For this review, take the finished solid that the model builds, in its own axes (mm). Face numbers are marked on the shaded views. A direction names the side the tool comes from. Give positions to 0.01 mm unless a question says otherwise; leave off trailing zeros. Order: outer loops, then holes, each group sorted by start corner. A loop starts at its lowest first (then second) coordinate and runs counter-clockwise, first axis right, second up.
Item 1: Consider section B-B (x = 0). Give the boundary of the cut face in (y, z), plus the area to 3 significant figures.
Item 2: For P1, Ø4, axis at x = -18.5, z = 0, coming from the -Y side; P2, Ø8, axis at x = 18.5, z = 0, coming from the +Y side; P3, Ø5, axis at x = -12, y = 4.5, coming from the -Z side; P4, Ø1, axis at y = 4, z = -4, coming from the +X side, all flat-tipped, find the tip position at first contact; note any pin that passes through.
Item 3: Consider section C-C (y = 0.5). Give the boundary of the cut face in (x, z).
Item 4: For probe 1 along Z at (x, y) = (0, 4.5); probe 2 along X at (y, z) = (1.25, 0.25); probe 3 along X at (y, z) = (7.5, -5.75), list the stretches that pass through material, from the lowest coordinate up.
Item 5: Consider section D-D (y = 6.25). Give the boundary of the cut face in (x, z), plus the area to 3 significant figures.
Item 6: Consider section A-A (z = 0). Give the boundary of the cut face in (x, y), plus the area to 3 significant figures.
Item 7: Machinability: for the marked faces 1 and 2, which of the approach directions +Z, -Z, +X, -X, +Y, -Y give a long, thin tool a straight path to every point of the face, cutting with its end or side? Answer none if there is none.
Autodesk Inventor part; units mm, degrees
ref_plane "YZ Plane" through (0, 0, 0) normal (1, 0, 0) x (0, 1, 0)
ref_plane "XZ Plane" through (0, 0, 0) normal (0, 1, 0) x (-1, 0, 0)
ref_plane "XY Plane" through (0, 0, 0) normal (0, 0, 1) x (1, 0, 0)
sketch "Sketch1" plane through (0, 0, 0) normal (0, 1, 0) x (-1, 0, 0)
  circle A0 centre (0, 0) radius 13.25
  circle A1 centre (0, 0) radius 4
  dimension "d0" = 26.5
  dimension "d1" = 8
extrude "Extrusion1" add sketch "Sketch1" along normal blind 8.5
sketch "Sketch2" plane through (0, 0, 0) normal (0, -1, 0) x (1, 0, 0)
  circle A0 centre (18.5, 0) radius 2.5
  circle A1 centre (-18.5, 0) radius 2.5
  circle A2 centre (18.5, 0) radius 5.25
  circle A3 centre (-18.5, 0) radius 5.25
  line L0 (20.7703, -4.7337) -> (5.7297, -11.9471)
  circle A4 centre (0, 0) radius 13.25
  line L1 (20.7703, 4.7337) -> (5.7297, 11.9471)
  line L2 (-5.7297, -11.9471) -> (-20.7703, -4.7337)
  line L3 (-5.7297, 11.9471) -> (-20.7703, 4.7337)
  point P0 (0, 18.5)
  point P1 (0, -18.5)
  dimension "d6" = 5
  dimension "d7" = 5
  dimension "d8" = 37
  dimension "d9" = 18.5
  dimension "d10" = 10.5
  dimension "d11" = 10.5
  dimension "d14" = 47.5
extrude "Extrusion2" add sketch "Sketch2" against normal blind 4.5 contours A2 | A2 A4 L1 | L0 A4 A2 | A4 A3 L3 | L2 A3 A4 | A3
properties part number "O_Do_Lan" material "Aluminum 6061-AHC"
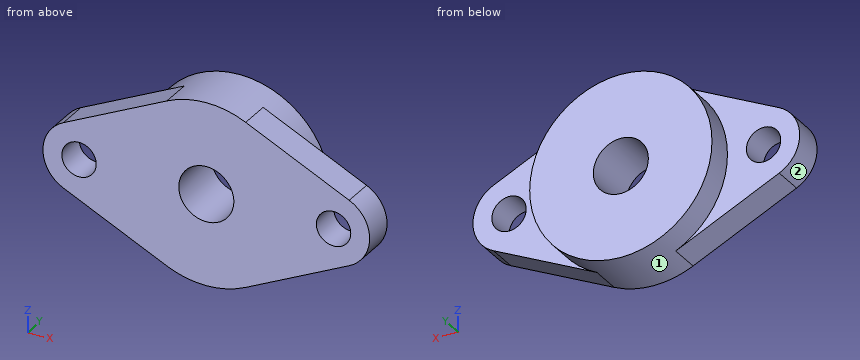
Resolved:
1. outline: (0, -13.25) - (8.5, -13.25) - (8.5, -4) - (0, -4) - close; (0, 4) - (8.5, 4) - (8.5, 13.25) - (0, 13.25) - close
1. area: 157 mm2
2. P1: passes through
2. P2: stops at y = 4.5
2. P3: stops at z = -10.14
2. P4: stops at x = 22.41
3. outline: (-20.77, -4.73) - (-5.73, -11.95) arc R13.25 ccw to (5.73, -11.95) - (20.77, -4.73) arc R5.25 ccw to (20.77, 4.73) - (5.73, 11.95) arc R13.25 ccw to (-5.73, 11.95) - (-20.77, 4.73) arc R5.25 ccw to start; hole circle Ø5 at (-18.5, 0); hole circle Ø8 at (0, 0); hole circle Ø5 at (18.5, 0)
4. probe 1: z = -13.25 to -4, 4 to 13.25
4. probe 2: x = -23.74 to -20.99, -16.01 to -3.99, 3.99 to 16.01, 20.99 to 23.74
4. probe 3: x = -11.94 to 11.94
5. outline: circle Ø26.5 at (0, 0); hole circle Ø8 at (0, 0)
5. area: 501 mm2
6. outline: (-23.75, 0) - (-21, 0) - (-21, 4.5) - (-23.75, 4.5) - close; (-16, 0) - (-4, 0) - (-4, 8.5) - (-13.25, 8.5) - (-13.25, 4.5) - (-16, 4.5) - close; (4, 0) - (16, 0) - (16, 4.5) - (13.25, 4.5) - (13.25, 8.5) - (4, 8.5) - close; (21, 0) - (23.75, 0) - (23.75, 4.5) - (21, 4.5) - close
6. area: 207 mm2
7. face 1: +Y
7. face 2: -X, +Y, -Y
